Verification items for the finished model (mm, model axes). A direction names the side the tool comes from. Round coordinates to 2 decimals unless told otherwise and drop trailing zeros. Loops run counter-clockwise (first coordinate to the right, second up) from the corner with the lowest first, then second, coordinate; pieces in that order, holes last. Notation, with made-up numbers: (8, 1.25) -> (20, 1.25) arc R22 cw to (20, 25.25) -> close; hole circle Ø7 at (-34.75, 17). An arc over 180 degrees is marked (long way). Write item = value, one per line.
```python
from build123d import *

# Parameters (mm, degrees)
ESQUISSE1_W             = 45
ESQUISSE1_H             = 250
BOSS_EXTRU_1_DEPTH      = 5
ESQUISSE2_W             = 80
ESQUISSE2_H             = 250
BOSS_EXTRU_2_DEPTH      = 5
ESQUISSE4_W             = 85
ESQUISSE4_H             = 250
BOSS_EXTRU_4_DEPTH      = 5
ESQUISSE5_R             = 5
ENL_V_MAT_EXTRU_1_DEPTH = 181


with BuildPart() as part:
    # Esquisse1 → Boss.-Extru.1 (new body)
    with BuildSketch(Plane.XY):
        with Locations((-22.5, 125)):
            Rectangle(ESQUISSE1_W, ESQUISSE1_H)
    boss_extru_1 = extrude(amount=BOSS_EXTRU_1_DEPTH)

    # Esquisse2 → Boss.-Extru.2 (add)
    with BuildSketch(Plane(origin=(0, 0, 0), x_dir=(0, 0, -1), z_dir=(1, 0, 0))):
        with Locations((35, 125)):
            Rectangle(ESQUISSE2_W, ESQUISSE2_H)
    boss_extru_2 = extrude(amount=BOSS_EXTRU_2_DEPTH)

    # Esquisse4 → Boss.-Extru.4 (add)
    with BuildSketch(Plane(origin=(0, 0, -75), x_dir=(-1, 0, 0), z_dir=(0, 0, -1))):
        with Locations((-42.5, 125)):
            Rectangle(ESQUISSE4_W, ESQUISSE4_H)
    boss_extru_4 = extrude(amount=BOSS_EXTRU_4_DEPTH)

    # Symétrie1: Boss.-Extru.1, Boss.-Extru.2, Boss.-Extru.4 across plane
    add(boss_extru_1.mirror(Plane(origin=(-45, 0, 5), x_dir=(0, 0, 1), z_dir=(1, 0, 0))))
    add(boss_extru_2.mirror(Plane(origin=(-45, 0, 5), x_dir=(0, 0, 1), z_dir=(1, 0, 0))))
    add(boss_extru_4.mirror(Plane(origin=(-45, 0, 5), x_dir=(0, 0, 1), z_dir=(1, 0, 0))))

    # Esquisse5 → Enlèv. mat.-Extru.1 (cut, through all)
    with BuildSketch(Plane(origin=(5, 0, 0), x_dir=(0, 0, -1), z_dir=(1, 0, 0))):
        with Locations((25.5, 125)):
            Circle(ESQUISSE5_R)
        with Locations((25.5, 200)):
            Circle(ESQUISSE5_R)
        with Locations((25.5, 50)):
            Circle(ESQUISSE5_R)
    extrude(amount=-ENL_V_MAT_EXTRU_1_DEPTH, mode=Mode.SUBTRACT)


solid = part.part
```
(1) Sectioned sample at C-C, the plane z = -44. Record the cut outline in (x, y).
Filled sheet:
outline = (-95, 0) -> (-90, 0) -> (-90, 250) -> (-95, 250) -> close; (0, 0) -> (5, 0) -> (5, 250) -> (0, 250) -> close
(2) Set-up check for faces 5 (the face through (-95, 127, -34)), 6 (the face through (46, 127, -75)), 7 (the face through (-90, 123, -39)): record each of +Z, -Z, +X, -X, +Y, -Y from which the full face is reachable in a straight line by a thin tool's end or side.
Filled sheet:
face_5 = +Z, -X, +Y, -Y
face_6 = +Z, +X, +Y, -Y
face_7 = -Z, +Y, -Y
(3) Sectioned sample at D-D, the plane x = -137. Record the cut outline in (y, z), and give its area (3 significant figures).
Filled sheet:
outline = (0, -80) -> (250, -80) -> (250, -75) -> (0, -75) -> close
area = 1,250 mm2
(4) Material ranges on probe 1 along Y at (x, z) = (-92, -25); probe 2 along X at (y, z) = (115, -23.5); probe 3 along Z at (x, y) = (73, 27), recorded low to high. Write a range as from..to.
Filled sheet:
probe_1 = 0..45.03, 54.97..120.03, 129.97..195.03, 204.97..250
probe_2 = -95..-90, 0..5
probe_3 = -80..-75
(5) Sectioned sample at B-B, the plane z = -25.5. Count the separate pieces of the cut face and the enclosed holes in it, and give its area (3 significant figures).
Filled sheet:
separate_pieces = 8
enclosed_holes = 0
area = 2,200 mm2
(6) Go/stop test with flat-tipped pins: pin 1 Ø9 at (y, z) = (50, -25.5) entering from +X; pin 2 Ø24 at (x, y) = (28.5, 170.5) entering from +Z; pin 3 Ø12 at (y, z) = (104.5, -6.5) entering from +X; pin 4 Ø16 at (y, z) = (125, -25.5) entering from -X. Record where each tip stops, or that it passes through.
Filled sheet:
pin_1 = through
pin_2 = -75
pin_3 = 5
pin_4 = -95
(7) Sectioned sample at A-A, the plane y = 125. Record the cut outline in (x, z), and give its area (3 significant figures).
Filled sheet:
outline = (-175, -80) -> (-90, -80) -> (-90, -30.5) -> (-95, -30.5) -> (-95, -75) -> (-175, -75) -> close; (-95, -20.5) -> (-90, -20.5) -> (-90, 0) -> (0, 0) -> (0, -20.5) -> (5, -20.5) -> (5, 5) -> (-95, 5) -> close; (0, -80) -> (85, -80) -> (85, -75) -> (5, -75) -> (5, -30.5) -> (0, -30.5) -> close
area = 2,000 mm2
(8) Draft check along X on faces 1 (the face through (5, 127, -34)), 2 (the face through (-44, 127, 0)), 3 (the face through (0, 123, -39)), 4 (the face through (2.535, 204.957, -24.849)). Enter one of: released by +X, released by -X, zero draft, split by the parting line, or undercut.
Filled sheet:
face_1 = released by +X
face_2 = undercut
face_3 = undercut
face_4 = zero draft
